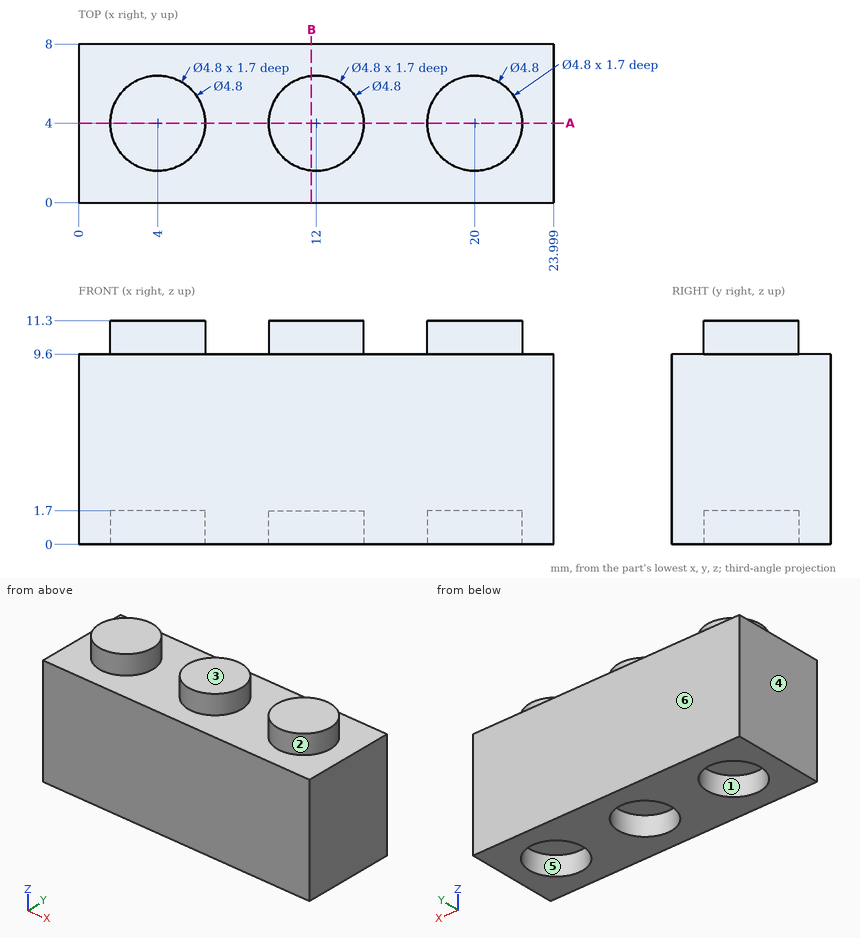
Here's the drawing with two shaded views (mm, measured from the low corner). I have some questions. A direction names the side the tool comes from. Give positions to 0.01 mm unless a question says otherwise; leave off trailing zeros. Loops run counter-clockwise (first coordinate to the right, second up) from the corner with the lowest first, then second, coordinate; pieces in that order, holes last. Notation, with made-up numbers: (63.5, 49.5) -> (67.5, 49.5) arc R8 cw to (67.5, 61.5) -> close; hole circle Ø3 at (-9, 61). An arc over 180 degrees is marked (long way). One line per item, written item: value.
Q1. I'm going to push a flat-ended pin straight in: pin 1 Ø3 at (x, y) = (4, 4) entering from -Z. Where does the tip first touch, or does it pass through?
Answers follow:
pin 1: z = 1.7
Q2. On a 3-axis mill with a long thin cutter (end or side, diameter ignored), from which of +Z, -Z, +X, -X, +Y, -Y can I reach the whole of each face in a straight line? I mean the marked faces 1, 2 and 3. Say none if no direction works.
Answers follow:
face 1: -Z
face 2: +Z
face 3: +Z, +X, -X, +Y, -Y
Q3. If I drill on line 1 along Y through (x, z) = (4, 1.05); line 2 along Z through (x, y) = (20, 1.5); line 3 along Z through (x, y) = (10.25, 5.5), over which ranges is the centre line in solid material (lowest first)?
Answers follow:
line 1: 0 to 1.6, 6.4 to 8
line 2: 0 to 9.6
line 3: 1.7 to 11.3
Q4. Suppose I cut it at B-B on x = 11.75. Please give me the cut outline in (y, z).
Answers follow:
outline: (0, 0) -> (1.61, 0) -> (1.61, 1.7) -> (6.39, 1.7) -> (6.39, 0) -> (8, 0) -> (8, 9.6) -> (6.39, 9.6) -> (6.39, 11.3) -> (1.61, 11.3) -> (1.61, 9.6) -> (0, 9.6) -> close
Q5. We'd pull the mould along Y, two halves only. Please class the marked faces 4, 5 and 6: pulls with the +Y half, pulls with the -Y half, needs draft (parallel to the pull), parting line crosses it, or undercut.
Answers follow:
face 4: needs draft
face 5: undercut
face 6: pulls with the +Y half
Q6. Suppose I cut it at A-A on y = 4. Please give me the cut outline in (x, z).
Answers follow:
outline: (0, 0) -> (1.6, 0) -> (1.6, 1.7) -> (6.4, 1.7) -> (6.4, 0) -> (9.6, 0) -> (9.6, 1.7) -> (14.4, 1.7) -> (14.4, 0) -> (17.6, 0) -> (17.6, 1.7) -> (22.4, 1.7) -> (22.4, 0) -> (24, 0) -> (24, 9.6) -> (22.4, 9.6) -> (22.4, 11.3) -> (17.6, 11.3) -> (17.6, 9.6) -> (14.4, 9.6) -> (14.4, 11.3) -> (9.6, 11.3) -> (9.6, 9.6) -> (6.4, 9.6) -> (6.4, 11.3) -> (1.6, 11.3) -> (1.6, 9.6) -> (0, 9.6) -> close
